```python
from build123d import *

# Parameters (mm, degrees)
BOSS_EXTRUDE1_DEPTH        = 101.6
F_7_0_201_DIAMETER_HOLE1_D = 5.1054
SKETCH5_R                  = 4.064
CUT_EXTRUDE2_DEPTH         = 128.476941935
SKETCH9_R                  = 3.81
CUT_EXTRUDE3_DEPTH         = 38.1


with BuildPart() as part:
    # Sketch1 → Boss-Extrude1 (new body)
    with BuildSketch(Plane.XY):
        Polygon((0, 0), (62.865, 0), (62.865, 44.45), (53.34, 44.45), (53.34, 20.32), (9.525, 20.32), (9.525, 44.45), (0, 44.45), align=None)
    extrude(amount=BOSS_EXTRUDE1_DEPTH)

    # #7 (0.201) Diameter Hole1 (through all)
    with Locations(Plane.ZY):
        with Locations((25.4, 34.29), (76.2, 34.29)):
            Hole(F_7_0_201_DIAMETER_HOLE1_D / 2)

    # Sketch5 → Cut-Extrude2 (cut, through all)
    with BuildSketch(Plane.ZY):
        with Locations((76.2, 12.7)):
            Circle(SKETCH5_R)
    extrude(amount=-CUT_EXTRUDE2_DEPTH, mode=Mode.SUBTRACT)

    # Sketch9 → Cut-Extrude3 (cut)
    with BuildSketch(Plane(origin=(0, 0, 0), x_dir=(-1, 0, 0), z_dir=(0, 0, -1))):
        with Locations((-31.4325, 12.7)):
            Circle(SKETCH9_R)
    extrude(amount=-CUT_EXTRUDE3_DEPTH, mode=Mode.SUBTRACT)


solid = part.part
```
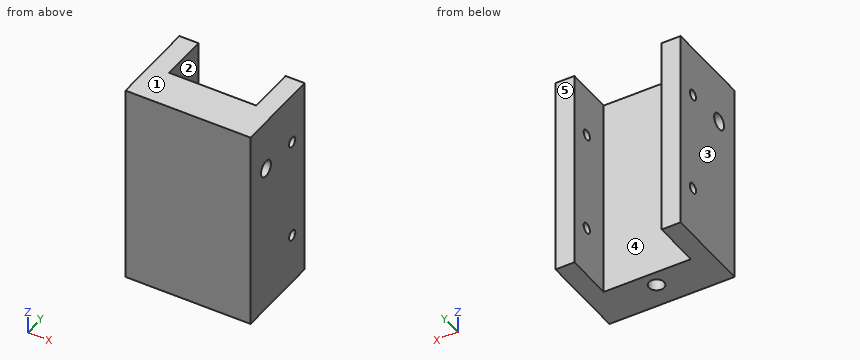
CAD build for the part. Positions are in the model's coordinates, mm. Face numbers are marked on the shaded views. A direction names the side the tool comes from. Round coordinates to 2 decimals unless told otherwise and drop trailing zeros. Order: outer loops, then holes, each group sorted by start corner. A loop starts at its lowest first (then second) coordinate and runs counter-clockwise, first axis right, second up. Notation, with made-up numbers: (89.5, 23.5) -> (141.5, 23.5) arc R18 ccw to (141.5, 45.5) -> close; hole circle Ø8 at (66, 73). An arc over 180 degrees is marked (long way). Write item = value, one per line.
(1) Flat gauge pins, fed straight in: P1, Ø10, axis at y = 36, z = 40, coming from the -X side; P2, Ø3, axis at x = 39.5, z = 60.5, coming from the +Y side; P3, Ø4.5, axis at y = 34.29, z = 25.4, coming from the -X side; P4, Ø6, axis at x = 31.43, y = 12.7, coming from the -Z side. Where does each tip first touch, or does it go through?
Answers follow:
P1 = 0
P2 = 20.32
P3 = through
P4 = 38.1
(2) Cut at B-B (y = 34.29). Write the cut outline in (x, z) (3 decimals).
Answers follow:
outline = (0, 0) -> (9.525, 0) -> (9.525, 22.847) -> (0, 22.847) -> close; (0, 27.953) -> (9.525, 27.953) -> (9.525, 73.647) -> (0, 73.647) -> close; (0, 78.753) -> (9.525, 78.753) -> (9.525, 101.6) -> (0, 101.6) -> close; (53.34, 0) -> (62.865, 0) -> (62.865, 22.847) -> (53.34, 22.847) -> close; (53.34, 27.953) -> (62.865, 27.953) -> (62.865, 73.647) -> (53.34, 73.647) -> close; (53.34, 78.753) -> (62.865, 78.753) -> (62.865, 101.6) -> (53.34, 101.6) -> close
(3) Pull direction X, two halves, no side cores. Call the marked faces 1, 2 and 3: +X half, -X half, draft (parallel to the pull), parting line (faces both ways), or undercut.
Answers follow:
face_1 = draft
face_2 = undercut
face_3 = -X half
(4) Cut at A-A (z = 25.4). State how many separate pieces and enclosed holes the cut face has, plus the area to 3 significant figures.
Answers follow:
separate_pieces = 3
enclosed_holes = 1
area = 1,590 mm²
(5) 3-axis set-ups, long thin cutter, end or side, ignore diameter. For the marked faces 4 and 5: which of +Z, -Z, +X, -X, +Y, -Y reach the whole face in a straight line?
Answers follow:
face_4 = +Z, -Z, +Y
face_5 = +Z, -Z, +X, -X, +Y
(6) Cut at D-D (z = 76.2). Write the cut outline in (x, y) (3 decimals).
Answers follow:
outline = (0, 0) -> (62.865, 0) -> (62.865, 8.636) -> (0, 8.636) -> close; (0, 16.764) -> (62.865, 16.764) -> (62.865, 31.737) -> (53.34, 31.737) -> (53.34, 20.32) -> (9.525, 20.32) -> (9.525, 31.737) -> (0, 31.737) -> close; (0, 36.843) -> (9.525, 36.843) -> (9.525, 44.45) -> (0, 44.45) -> close; (53.34, 36.843) -> (62.865, 36.843) -> (62.865, 44.45) -> (53.34, 44.45) -> close
(7) Cut at C-C (x = 6.5). Write the cut outline in (y, z).
Answers follow:
outline = (0, 0) -> (44.45, 0) -> (44.45, 101.6) -> (0, 101.6) -> close; hole circle Ø8.13 at (12.7, 76.2); hole circle Ø5.11 at (34.29, 25.4); hole circle Ø5.11 at (34.29, 76.2)
(8) Drill centre lines: L1, parallel to Z at x = 4, y = 34; L2, parallel to X at y = 40, z = 75.5 (3 decimals); L3, parallel to Y at x = 27, z = 58. Where is each one in solid material? Low to high.
Answers follow:
L1 = 0 to 22.86, 27.94 to 73.66, 78.74 to 101.6
L2 = 0 to 9.525, 53.34 to 62.865
L3 = 0 to 20.32
